The listing builds one solid part. Answer for the finished solid, in the listing's coordinates (mm). A direction names the side the tool comes from. Round coordinates to 2 decimals unless told otherwise and drop trailing zeros. Write each loop counter-clockwise with the first axis right and the second up, starting at its lowest first coordinate (ties: lowest second). Pieces come first, ordered by that corner, then holes.
from build123d import *

# Parameters (mm, degrees)
SKETCH_1_R      = 1.6
EXTRUDE_1_DEPTH = 3
FILLET_1_R      = 60
FILLET_2_R      = 2
FILLET_3_R      = 20
FILLET_4_R      = 2


with BuildPart() as part:
    # ｽｹｯﾁ1 → ﾎﾞｽ - 押し出し1 (new body)
    with BuildSketch(Plane.XY):
        Polygon((-30, 0), (0, 0), (0, 30), (-17.573593129, 30), (-35, 47.426406871), (-35, 199.644660941), (-24.644660941, 210), (0, 210), (0, 240), (-30, 240), (-95, 175), (-95, 65), align=None)
        Polygon((-75, 159.644660941), (-45, 189.644660941), (-45, 130.035533906), (-75, 130.035533906), align=None, mode=Mode.SUBTRACT)
        Polygon((-45, 120.035533906), (-45, 57.426406871), (-75, 87.426406871), (-75, 120.035533906), align=None, mode=Mode.SUBTRACT)
        with Locations((-90, 66)):
            Circle(SKETCH_1_R, mode=Mode.SUBTRACT)
        with Locations((-31.514718626, 10)):
            Circle(SKETCH_1_R, mode=Mode.SUBTRACT)
        with Locations((-5, 4)):
            Circle(SKETCH_1_R, mode=Mode.SUBTRACT)
        with Locations((-5, 225)):
            Circle(SKETCH_1_R, mode=Mode.SUBTRACT)
        with Locations((-40, 125.035533906)):
            Circle(SKETCH_1_R, mode=Mode.SUBTRACT)
    extrude(amount=EXTRUDE_1_DEPTH)

    # ﾌｨﾚｯﾄ1
    fillet_1_edges = [part.edges().sort_by_distance(p)[0] for p in [
        (-75, 159.644660941, 1.5),
        (-95, 175, 1.5),
        (-30, 240, 1.5),
        (-75, 87.426406871, 1.5),
    ]]
    fillet(fillet_1_edges, radius=FILLET_1_R)

    # ﾌｨﾚｯﾄ2
    fillet_2_edges = [part.edges().sort_by_distance(p)[0] for p in [
        (-17.573593129, 30, 1.5),
        (0, 30, 1.5),
        (0, 0, 1.5),
        (0, 240, 1.5),
        (0, 210, 1.5),
        (-24.644660941, 210, 1.5),
        (-35, 199.644660941, 1.5),
        (-35, 47.426406871, 1.5),
    ]]
    fillet(fillet_2_edges, radius=FILLET_2_R)

    # ﾌｨﾚｯﾄ3
    fillet_3_edges = [part.edges().sort_by_distance(p)[0] for p in [
        (-30, 0, 1.5),
        (-95, 65, 1.5),
    ]]
    fillet(fillet_3_edges, radius=FILLET_3_R)

    # ﾌｨﾚｯﾄ4
    fillet_4_edges = [part.edges().sort_by_distance(p)[0] for p in [
        (-45, 189.644660941, 1.5),
        (-75, 130.035533906, 1.5),
        (-45, 130.035533906, 1.5),
        (-75, 120.035533906, 1.5),
        (-45, 57.426406871, 1.5),
        (-45, 120.035533906, 1.5),
    ]]
    fillet(fillet_4_edges, radius=FILLET_4_R)


solid = part.part
1. Section C-C on x = -55 is taken. Determine the outline of the cut face in (y, z), plus the area to 3 significant figures.
Geometry says:
outline: (25, 0) - (67.43, 0) - (67.43, 3) - (25, 3) - close; (120.04, 0) - (130.04, 0) - (130.04, 3) - (120.04, 3) - close; (179.64, 0) - (215, 0) - (215, 3) - (179.64, 3) - close
area: 263 mm2
2. A tool of negligible diameter and unlimited length cuts with its end or side. For faces 1 (the face through (-29.27, 1.48, 1.52)), 2 (the face through (-26.173, 38.599, 1.479)), 3 (the face through (-70.558, 157.448, 1.521)), from which of +Z, -Z, +X, -X, +Y, -Y can it reach the whole face along a straight path? Write none if from no direction.
Geometry says:
face 1: +Z, -Z, -X, -Y
face 2: +Z, -Z, +X
face 3: +Z, -Z
3. Section B-B on y = 170.5 is taken. Determine the outline of the cut face in (x, z).
Geometry says:
outline: (-91.44, 0) - (-63.22, 0) - (-63.22, 3) - (-91.44, 3) - close; (-45, 0) - (-35, 0) - (-35, 3) - (-45, 3) - close
4. Given pin 1 (2.5 mm diameter, centred on x = -31.51, y = 10, fed in from -Z); pin 2 (0.9 mm diameter, centred on x = -6, z = 1, fed in from +Y); pin 3 (0.9 mm diameter, centred on y = 93, z = 1, fed in from +X); pin 4 (0.9 mm diameter, centred on x = -64, z = 1.5, fed in from +Y), each flat-ended and moving along its own axis, determine where each tip first touches the part or whether it passes through.
Geometry says:
pin 1: passes through
pin 2: stops at y = 240
pin 3: stops at x = -35
pin 4: stops at y = 206.45
5. Section D-D on z = 1.1 is taken. Give the number of separate pieces and of enclosed holes in the cut face, plus the area to 3 significant figures.
Geometry says:
separate pieces: 1
enclosed holes: 7
area: 9,670 mm2
6. For a pull along X with two mould halves and no side action, classify faces 4 (the face through (-93.435, 65.529, 1.521)), 5 (the face through (-29.887, 204.758, 1.479)), 6 (the face through (-52.857, 65.284, 1.479)) as released by +X, released by -X, zero draft, split by the parting line, or undercut.
Geometry says:
face 4: released by -X
face 5: released by +X
face 6: undercut
7. Section A-A on x = -27.5 is taken. Determine the outline of the cut face in (y, z).
Geometry says:
outline: (0.85, 0) - (39.93, 0) - (39.93, 3) - (0.85, 3) - close; (207.14, 0) - (235.68, 0) - (235.68, 3) - (207.14, 3) - close
8. Straight lines are drawn through the part: line 1 along Y through (x, z) = (-5, 1.25); line 2 along Y through (x, z) = (-62, 1.2); line 3 along Y through (x, z) = (-32.5, 2.6). For each, find the intervals that lie inside material, in ascending order.
Geometry says:
line 1: y = 0 to 2.4, 5.6 to 30, 210 to 223.4, 226.6 to 240
line 2: y = 32 to 74.98, 120.04 to 130.04, 172.09 to 208
line 3: y = 3.16 to 8.74, 11.26 to 44.93, 202.14 to 233.4
